Build history of the part. All positions in model axes, mm. Face numbers are marked on the shaded views. Coordinates: 2 decimals unless noted, no trailing zeros. Loops run counter-clockwise (first coordinate to the right, second up) from the corner with the lowest first, then second, coordinate; pieces in that order, holes last. Notation, with made-up numbers: (55, 37.25) - (90, 37.25) arc R25 cw to (90, 53.25) - close; hole circle Ø11 at (54, 36). An arc over 180 degrees is marked (long way). One line per item, written item: value.
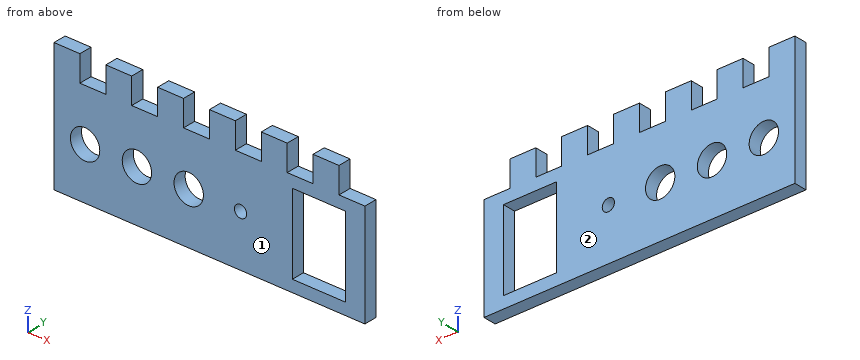
```python
from build123d import *

# Parameters (mm, degrees)
SKETCH1_R           = 3.6
SKETCH1_R_2         = 1.5
SKETCH1_W           = 13
SKETCH1_H           = 19.6
BOSS_EXTRUDE1_DEPTH = 3.175


with BuildPart() as part:
    # Sketch1 → Boss-Extrude1 (new body)
    with BuildSketch(Plane(origin=(0, 0, 0), x_dir=(1, 0, 0), z_dir=(0, 1, 0))):
        Polygon((0, 0), (0, -6.35), (6.35, -6.35), (6.35, 0), (12.7, 0), (12.7, -6.35), (19.05, -6.35), (19.05, 0), (25.4, 0), (25.4, -6.35), (31.75, -6.35), (31.75, 0), (38.1, 0), (38.1, -6.35), (44.45, -6.35), (44.45, 0), (50.8, 0), (50.8, -6.35), (57.15, -6.35), (57.15, 0), (63.5, 0), (63.5, -6.35), (69.85, -6.35), (69.85, 0), (76.2, 0), (76.2, 25.4), (0, 25.4), align=None)
        with Locations(Location((7.62, 12.7, 0), (0, 0, 270))):
            Circle(SKETCH1_R, mode=Mode.SUBTRACT)
        with Locations(Location((20.32, 12.7, 0), (0, 0, 270))):
            Circle(SKETCH1_R, mode=Mode.SUBTRACT)
        with Locations(Location((33.02, 12.7, 0), (0, 0, 270))):
            Circle(SKETCH1_R, mode=Mode.SUBTRACT)
        with Locations(Location((45.72, 12.7, 0), (0, 0, 270))):
            Circle(SKETCH1_R_2, mode=Mode.SUBTRACT)
        with Locations((64.92, 12.7)):
            Rectangle(SKETCH1_W, SKETCH1_H, mode=Mode.SUBTRACT)
    extrude(amount=BOSS_EXTRUDE1_DEPTH)


solid = part.part
```
Item 1: Cut at C-C, the plane y = 1.7. Give the number of separate pieces and of enclosed holes in the cut face, then the cut area to 3 significant figures.
Check result:
separate pieces: 1
enclosed holes: 5
area: 1,790 mm^2
Item 2: Pull direction Y, two halves, no side cores. Call the marked faces 1 and 2: released by +Y, released by -Y, zero draft, split by the parting line, or undercut.
Check result:
face 1: released by -Y
face 2: released by +Y
Item 3: Cut at D-D, the plane x = 45.72. Write the cut outline in (y, z) (3 decimals).
Check result:
outline: (0, -25.4) - (3.175, -25.4) - (3.175, -14.2) - (0, -14.2) - close; (0, -11.2) - (3.175, -11.2) - (3.175, 0) - (0, 0) - close
Item 4: Cut at A-A, the plane z = -12.7. Write the cut outline in (x, y) (3 decimals), then the cut area to 3 significant figures.
Check result:
outline: (0, 0) - (4.02, 0) - (4.02, 3.175) - (0, 3.175) - close; (11.22, 0) - (16.72, 0) - (16.72, 3.175) - (11.22, 3.175) - close; (23.92, 0) - (29.42, 0) - (29.42, 3.175) - (23.92, 3.175) - close; (36.62, 0) - (44.22, 0) - (44.22, 3.175) - (36.62, 3.175) - close; (47.22, 0) - (58.42, 0) - (58.42, 3.175) - (47.22, 3.175) - close; (71.42, 0) - (76.2, 0) - (76.2, 3.175) - (71.42, 3.175) - close
area: 123 mm^2
Item 5: Drop flat-ended pins along their axis: P1, Ø6.5, axis at x = 33.02, z = -12.7, coming from the +Y side; P2, Ø1, axis at x = 48, y = 1, coming from the +Z side. Give the stop position or say it passes through.
Check result:
P1: passes through
P2: stops at z = 0
Item 6: Cut at B-B, the plane x = 33.02. Write the cut outline in (y, z) (3 decimals), then the cut area to 3 significant figures.
Check result:
outline: (0, -25.4) - (3.175, -25.4) - (3.175, -16.3) - (0, -16.3) - close; (0, -9.1) - (3.175, -9.1) - (3.175, 0) - (0, 0) - close
area: 57.8 mm^2
Item 7: Probe probe 1 along X at (y, z) = (2.45, -12.7); probe 2 along Z at (x, y) = (61, 0.3); probe 3 along X at (y, z) = (2.05, -18.5). List the from-to ranges inside material, lowest first. Write a range as from..to.
Check result:
probe 1: x = 0..4.02, 11.22..16.72, 23.92..29.42, 36.62..44.22, 47.22..58.42, 71.42..76.2
probe 2: z = -25.4..-22.5, -2.9..0
probe 3: x = 0..58.42, 71.42..76.2
